Could you check a few things on this drawing? It's one solid part, dimensions in mm from its lowest x, y, z. Give positions to 0.01 mm unless a question says otherwise; leave off trailing zeros. Loops run counter-clockwise (first coordinate to the right, second up) from the corner with the lowest first, then second, coordinate; pieces in that order, holes last. Notation, with made-up numbers: M -32,66.5 L 19,66.5 A27 ccw 19,103.5 Z; hole C -2,11 d5. An arc over 180 degrees is marked long. Answer as CSV lines item,"result". Start each with the question number.
Item 1: Will these pins go through, and if not, where does the flat tip stop? P1, Ø1.5, axis at x = 5.5, y = 3, coming from the +Z side; P2, Ø7.5, axis at x = 7.14, z = 8.25, coming from the -Y side.
Item 2: I want a section at A-A on y = 0.45. List the corners of the cut face in (x, z) for me (1 decimal).
Item 3: If I drill on line 1 along Z through (x, y) = (6.25, 3.75) (1 decimal); line 2 along X through (y, z) = (4.05, 5) (1 decimal); line 3 along Z through (x, y) = (7.5, 4.75) (1 decimal), over which ranges is the centre line in solid material (lowest first)? Write a range as from..to.
Item 4: If we mould it in two halves opening along X, with no side actions, what happens to the marked faces 1, 2 and 3? For each: released by +X, released by -X, zero draft, split by the parting line, or undercut.
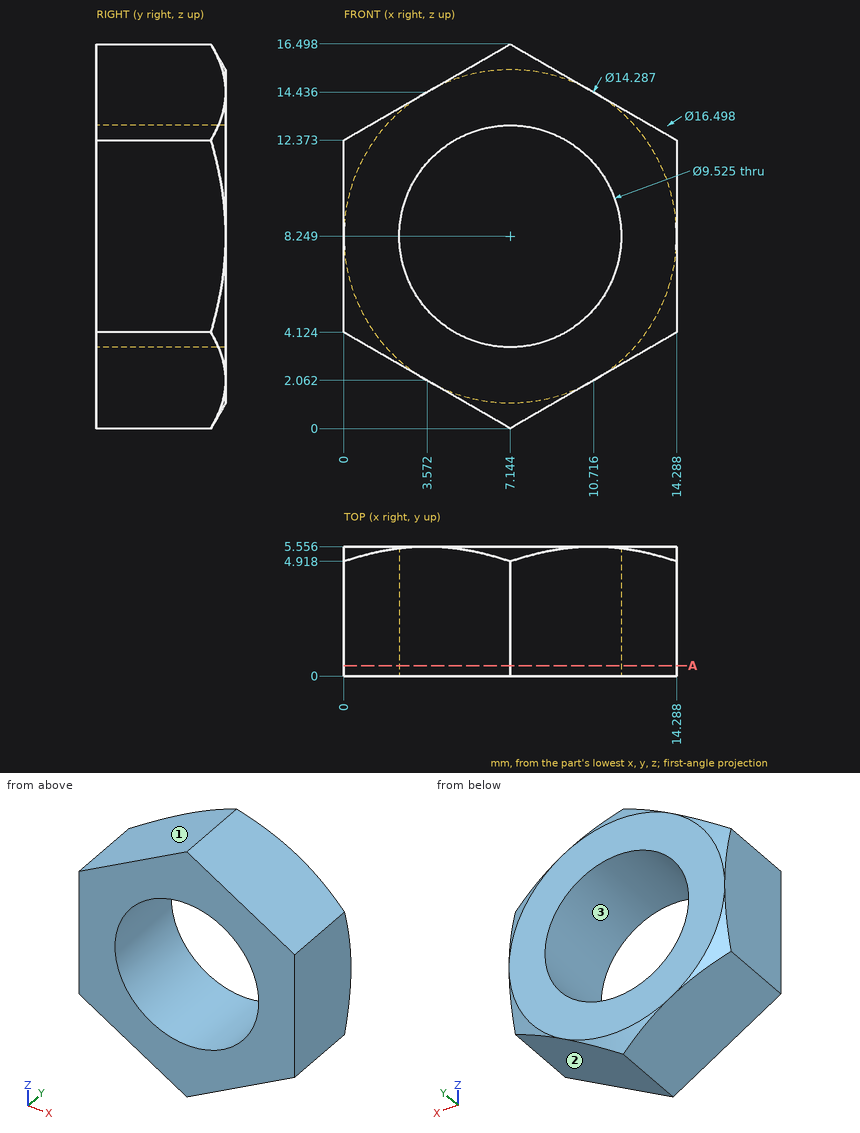
Result:
1,P1,"z = 15.98"
1,P2,"through"
2,outline,"M 0,4.1 L 7.1,0 L 14.3,4.1 L 14.3,12.4 L 7.1,16.5 L 0,12.4 Z; hole C 7.1,8.2 d9.5"
3,line 1,"0.5..3.6, 12.9..16"
3,line 2,"0..3.7, 10.6..14.3"
3,line 3,"0.2..3.5, 13..16.3"
4,face 1,"released by -X"
4,face 2,"released by +X"
4,face 3,"undercut"
